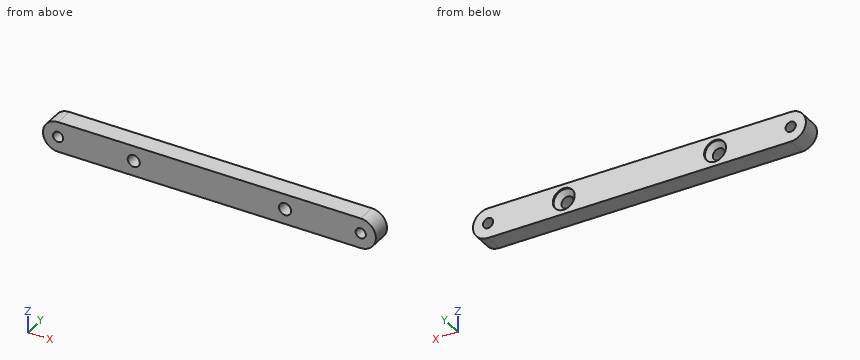
```python
from build123d import *

# Parameters (mm, degrees)
ESQUISSE1_R        = 1.35
BOSS_EXTRU_1_DEPTH = 5


with BuildPart() as part:
    # Esquisse1 → Boss.-Extru.1 (new body)
    with BuildSketch(Plane(origin=(0, 0, 0), x_dir=(1, 0, 0), z_dir=(0, 1, 0))):
        with BuildLine():
            Line((40, -4), (-40, -4))
            ThreePointArc((-40, -4), (-44, 0), (-40, 4))
            Line((-40, 4), (40, 4))
            ThreePointArc((40, 4), (44, 0), (40, -4))
        make_face()
        with Locations(Location((-40, 0, 0), (0, 0, 270))):
            Circle(ESQUISSE1_R, mode=Mode.SUBTRACT)
        with Locations(Location((40, 0, 0), (0, 0, 90))):
            Circle(ESQUISSE1_R, mode=Mode.SUBTRACT)
    extrude(amount=BOSS_EXTRU_1_DEPTH)

    # Esquisse2 → Fraisage pour vis à tête fraisée M31 (revolve, cut)
    with BuildSketch(Plane(origin=(-20, 5, 0), x_dir=(0, 0, 1), z_dir=(1, 0, 0))):
        Polygon((0, 0), (0, 5), (1.6, 5), (1.6, 1.7), (2.9, 0.4), (2.9, 0), align=None)
    fraisage_pour_vis_t_te_frais_e_m31 = revolve(axis=Axis((-20, 11.35, 0), (0, -1, 0)), mode=Mode.SUBTRACT)

    # Symétrie1: Fraisage pour vis à tête fraisée M31 across plane
    add(fraisage_pour_vis_t_te_frais_e_m31.mirror(Plane(origin=(0, 0, 0), x_dir=(0, 0, 1), z_dir=(1, 0, 0))), mode=Mode.SUBTRACT)


solid = part.part
```
The listing builds one solid part. Answer for the finished solid, in the listing's coordinates (mm). Coordinates: 2 decimals unless noted, no trailing zeros. Order: outer loops, then holes, each group sorted by start corner. A loop starts at its lowest first (then second) coordinate and runs counter-clockwise, first axis right, second up. Notation, with made-up numbers: M 40.25,13.5 L 84.25,13.5 A25 ccw 84.25,42.5 Z; hole C 53,17 d1. An arc over 180 degrees is marked long. Answer as a JSON object with one key per item and string values. Group by question number.
1. Section A-A on y = 2.15 is taken. Write down the section's boundary in (x, z), then the cut area to 3 significant figures.
2. Flat-ended cylindrical pins translate along their axes: P1, Ø4, axis at x = 20, z = 0, coming from the +Y side; P2, Ø4.5, axis at x = -20, z = 0, coming from the +Y side; P3, Ø1, axis at y = 4, z = 1, coming from the +X side. Find the tip coordinate at first contact, or state that the pin passes through.
3. Section C-C on x = -20 is taken. Write down the section's boundary in (y, z).
4. Straight lines are drawn through the part: line 1 (X direction, y = 0.95, z = 0); line 2 (Z direction, x = -20, y = 2.45); line 3 (X direction, y = 4.75, z = 0). For each, find the intervals that lie inside material, in ascending order.
5. Section B-B on z = 0 is taken. Write down the section's boundary in (x, y), then the cut area to 3 significant figures.
Values follow:
{
 "1": {"outline": "M -40,-4 L 40,-4 A4 ccw 40,4 L -40,4 A4 ccw Z; hole C -40,0 d2.7; hole C -20,0 d3.2; hole C 20,0 d3.2; hole C 40,0 d2.7", "area": "663 mm2"},
 "2": {"P1": "y = 3.7", "P2": "y = 3.95", "P3": "x = 43.97"},
 "3": {"outline": "M 0,-4 L 5,-4 L 5,-2.9 L 4.6,-2.9 L 3.3,-1.6 L 0,-1.6 Z; M 0,1.6 L 3.3,1.6 L 4.6,2.9 L 5,2.9 L 5,4 L 0,4 Z"},
 "4": {"line 1": "-44 to -41.35, -38.65 to -21.6, -18.4 to 18.4, 21.6 to 38.65, 41.35 to 44", "line 2": "-4 to -1.6, 1.6 to 4", "line 3": "-44 to -41.35, -38.65 to -22.9, -17.1 to 17.1, 22.9 to 38.65, 41.35 to 44"},
 "5": {"outline": "M -44,0 L -41.35,0 L -41.35,5 L -44,5 Z; M -38.65,0 L -21.6,0 L -21.6,3.3 L -22.9,4.6 L -22.9,5 L -38.65,5 Z; M -18.4,0 L 18.4,0 L 18.4,3.3 L 17.1,4.6 L 17.1,5 L -17.1,5 L -17.1,4.6 L -18.4,3.3 Z; M 21.6,0 L 38.65,0 L 38.65,5 L 22.9,5 L 22.9,4.6 L 21.6,3.3 Z; M 41.35,0 L 44,0 L 44,5 L 41.35,5 Z", "area": "376 mm2"}
}
